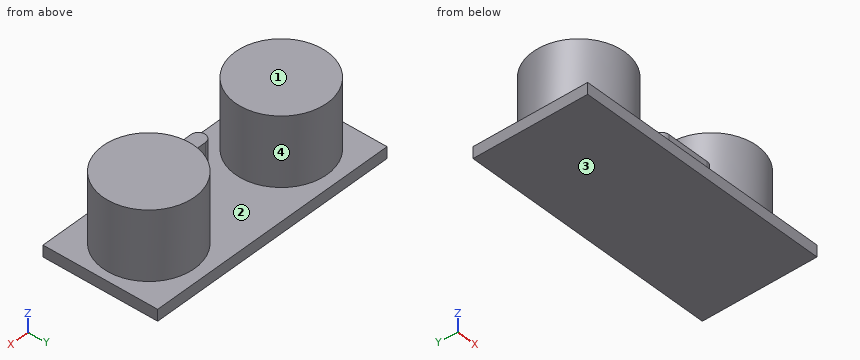
Autodesk Inventor part; units mm, degrees
ref_plane "YZ Plane" through (0, 0, 0) normal (1, 0, 0) x (0, 1, 0)
ref_plane "XZ Plane" through (0, 0, 0) normal (0, 1, 0) x (-1, 0, 0)
ref_plane "XY Plane" through (0, 0, 0) normal (0, 0, 1) x (1, 0, 0)
sketch "Esquisse1" plane through (0, 0, 0) normal (0, 0, 1) x (1, 0, 0)
  line L0 (0, 20) -> (45, 20)
  line L1 (45, 20) -> (45, 0)
  line L2 (45, 0) -> (0, 0)
  line L3 (0, 0) -> (0, 20)
  line L4 (-9, 0) -> (54, 0)
  line L5 (0, -4) -> (0, 24)
  point P0 (0, 0)
  dimension "d0" = 20
  dimension "d1" = 45
extrude "Extrusion1" add sketch "Esquisse1" along normal blind 2
sketch "Esquisse2" plane through (0, 0, 2) normal (0, 0, 1) x (1, 0, 0)
  circle A0 centre (9.5, 10) radius 8
  circle A1 centre (35.5, 10) radius 8
  line L0 (0, 10) -> (43.5, 10)
  line L1 (45, 20) -> (0, 20)
  line L2 (0, 20) -> (0, 0)
  dimension "d6" = 16
  dimension "d4" = 10
  dimension "d5" = 16
  dimension "d7" = 26
  dimension "d8" = 9.5
extrude "Extrusion2" add sketch "Esquisse2" along normal blind 12
sketch "Esquisse3" plane through (0, 0, 2) normal (0, 0, 1) x (1, 0, 0)
  line L0 (18.75, 3.75) -> (26.25, 3.75) construction
  line L1 (18.75, 2.5) -> (26.25, 2.5)
  line L2 (26.25, 5) -> (18.75, 5)
  arc A0 (18.75, 5) -> (18.75, 2.5) centre (18.75, 3.75) ccw
  arc A1 (26.25, 2.5) -> (26.25, 5) centre (26.25, 3.75) ccw
  line L3 (45, 0) -> (45, 20)
  line L4 (0, 0) -> (45, 0)
  point P0 (22.5, 3.75)
  point P1 (27.5, 3.75)
  point P2 (17.5, 3.75)
  dimension "d11" = 10
  dimension "d12" = 2.5
  dimension "d13" = 22.5
  dimension "d14" = 5
extrude "Extrusion3" add sketch "Esquisse3" along normal blind 4
equation "\"d6\" = d5"
properties part number "distance"
CAD build for the part. Positions are in the model's coordinates, mm. Face numbers are marked on the shaded views. A direction names the side the tool comes from. Coordinates: 2 decimals unless noted, no trailing zeros. Loops run counter-clockwise (first coordinate to the right, second up) from the corner with the lowest first, then second, coordinate; pieces in that order, holes last. Notation, with made-up numbers: (-4.75, 22.5) - (18.25, 22.5) arc R21 ccw to (18.25, 61.5) - close; hole circle Ø9 at (10, 54.5). An arc over 180 degrees is marked (long way). Write item = value, one per line. Start each with the question number.
Q1. Which spindle directions (+Z, -Z, +X, -X, +Y, -Y) get a long thin tool onto all of the face, cutting with end or side? Do the marked faces 3 and 4. Say none if no direction does.
Q2. Pull direction X, two halves, no side cores. Call the marked faces 1 and 2: pulls with the +X half, pulls with the -X half, needs draft (parallel to the pull), parting line crosses it, or undercut.
Q3. Flat gauge pins, fed straight in: pin 1 Ø1.5 at (x, z) = (8, 6) entering from +Y; pin 2 Ø8 at (y, z) = (12, 10) entering from +X; pin 3 Ø2 at (y, z) = (18, 12.5) entering from -X. Where does each tip first touch, or does it go through?
Q4. Cut at C-C, the plane y = 10. List the corners of the cut face in (x, z).
Q5. Cut at D-D, the plane z = 10.75. List the corners of the cut face in (x, y).
Q6. Cut at B-B, the plane x = 35.5. List the corners of the cut face in (y, z), then the cut area to 3 significant figures.
Q7. Cut at A-A, the plane z = 5. List the corners of the cut face in (x, y).
Q8. Drill centre lines: L1, parallel to X at y = 4, z = 4.25; L2, parallel to Z at x = 20, y = 14.5; L3, parallel to X at y = 10.5, z = 9.75. Where is each one in solid material? Low to high.
Computed:
q1.face_3 = -Z, +X, -X, +Y, -Y
q1.face_4 = +Z
q2.face_1 = needs draft
q2.face_2 = undercut
q3.pin_1 = 17.96
q3.pin_2 = 43.5
q3.pin_3 = 5.63
q4.outline = (0, 0) - (45, 0) - (45, 2) - (43.5, 2) - (43.5, 14) - (27.5, 14) - (27.5, 2) - (17.5, 2) - (17.5, 14) - (1.5, 14) - (1.5, 2) - (0, 2) - close
q5.outline = circle Ø16 at (9.5, 10); circle Ø16 at (35.5, 10)
q6.outline = (0, 0) - (20, 0) - (20, 2) - (18, 2) - (18, 14) - (2, 14) - (2, 2) - (0, 2) - close
q6.area = 232 mm²
q7.outline = circle Ø16 at (9.5, 10); (18.75, 2.5) - (26.25, 2.5) arc R1.25 ccw to (26.25, 5) - (18.75, 5) arc R1.25 ccw to start; circle Ø16 at (35.5, 10)
q8.L1 = 4.21 to 14.79, 17.53 to 27.47, 30.21 to 40.79
q8.L2 = 0 to 2
q8.L3 = 1.52 to 17.48, 27.52 to 43.48
